The model under review builds one solid part; all positions refer to its coordinate system, in mm. Face numbers are marked on the shaded views. A direction names the side the tool comes from. Coordinates: 2 decimals unless noted, no trailing zeros. Order: outer loops, then holes, each group sorted by start corner. A loop starts at its lowest first (then second) coordinate and runs counter-clockwise, first axis right, second up. Notation, with made-up numbers: M -6,3 L 31,3 A23 cw 31,32 Z; hole C 63.5,49.25 d5. An arc over 180 degrees is marked long. Answer in a Markdown table with one row per item.
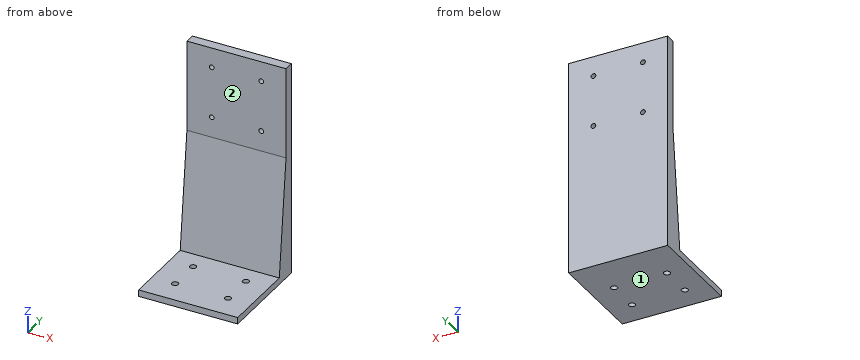
from build123d import *

# Parameters (mm, degrees)
F0_W     = 60
F0_H     = 60
F0_R     = 1.95
F1_DEPTH = 4
F2_W     = 60
F2_H     = 126
F2_R     = 1.45
F3_DEPTH = 6
F5_DEPTH = 60


with BuildPart() as f1:
    # F0 (on Top) → F1 (new body)
    with BuildSketch(Plane.XY):
        Rectangle(F0_W, F0_H)
        with Locations((-16, -15)):
            Circle(F0_R, mode=Mode.SUBTRACT)
        with Locations((16, -15)):
            Circle(F0_R, mode=Mode.SUBTRACT)
        with Locations((-16, 5)):
            Circle(F0_R, mode=Mode.SUBTRACT)
        with Locations((16, 5)):
            Circle(F0_R, mode=Mode.SUBTRACT)
    extrude(amount=F1_DEPTH)

    # F2 (on face) → F3 (join)
    with BuildSketch(Plane(origin=(0, 30, 0), x_dir=(-1, 0, 0), z_dir=(0, 1, 0))):
        with Locations((0, 67)):
            Rectangle(F2_W, F2_H)
        with Locations((-15, 87)):
            Circle(F2_R, mode=Mode.SUBTRACT)
        with Locations((-15, 118)):
            Circle(F2_R, mode=Mode.SUBTRACT)
        with Locations((15, 87)):
            Circle(F2_R, mode=Mode.SUBTRACT)
        with Locations((15, 118)):
            Circle(F2_R, mode=Mode.SUBTRACT)
    extrude(amount=-F3_DEPTH)

    # F4 (on face) → F5 (join)
    with BuildSketch(Plane.YZ.offset(30)):
        Polygon((24, 74.602762), (16.5, 4), (24, 4), align=None)
    extrude(amount=-F5_DEPTH)


solid = f1.part
(1) Take a section at B-B (z = 87). Write out the cut boundary in (x, y).
Report:
| item | result |
|---|---|
| outline | M -30,24 L -16.45,24 L -16.45,30 L -30,30 Z; M -13.55,24 L 13.55,24 L 13.55,30 L -13.55,30 Z; M 16.45,24 L 30,24 L 30,30 L 16.45,30 Z |
(2) To check wall thickness, follow line 1 (X direction, y = 28.6, z = 87); line 2 (Y direction, x = -16, z = 1.45); line 3 (Z direction, x = -15, y = 25). State the ranges of each line that lie inside material, in increasing order. Write a range as [from, to].
Report:
| item | result |
|---|---|
| line 1 | [-30, -16.45], [-13.55, 13.55], [16.45, 30] |
| line 2 | [-30, -16.95], [-13.05, 3.05], [6.95, 30] |
| line 3 | [0, 85.55], [88.45, 116.55], [119.45, 130] |
(3) Insertion check: P1, Ø3.5, axis at x = -16, y = 5, coming from the -Z side; P2, Ø1.5, axis at x = -3, z = 35.5, coming from the -Y side; P3, Ø3.5, axis at x = 15, z = 118, coming from the -Y side; P4, Ø10, axis at x = 5.5, z = 22, coming from the -Y side. Each pin has a flat end and moves straight along its axis. Give the tip position at first contact, or say it passes through.
Report:
| item | result |
|---|---|
| P1 | through |
| P2 | y = 19.77 |
| P3 | y = 24 |
| P4 | y = 17.88 |
(4) Take a section at A-A (y = 5). Write out the cut boundary in (x, z).
Report:
| item | result |
|---|---|
| outline | M -30,0 L -17.95,0 L -17.95,4 L -30,4 Z; M -14.05,0 L 14.05,0 L 14.05,4 L -14.05,4 Z; M 17.95,0 L 30,0 L 30,4 L 17.95,4 Z |
(5) Take a section at D-D (z = 40.5). Write out the cut boundary in (x, y).
Report:
| item | result |
|---|---|
| outline | M -30,20.38 L 30,20.38 L 30,30 L -30,30 Z |
(6) Take a section at C-C (x = -4). Write out the cut boundary in (y, z).
Report:
| item | result |
|---|---|
| outline | M -30,0 L 30,0 L 30,130 L 24,130 L 24,74.6 L 16.5,4 L -30,4 Z |
(7) Machinability: for the marked faces 1 and 2, which of the approach directions +Z, -Z, +X, -X, +Y, -Y give a long, thin tool a straight path to every point of the face, cutting with its end or side? Answer none if there is none.
Report:
| item | result |
|---|---|
| face 1 | -Z, +X, -X, +Y, -Y |
| face 2 | +Z, +X, -X, -Y |
